Source: CAD feature listing. Evaluate the final solid. Frame: model axes, mm. A direction names the side the tool comes from. Round coordinates to 2 decimals unless told otherwise and drop trailing zeros. Order: outer loops, then holes, each group sorted by start corner. A loop starts at its lowest first (then second) coordinate and runs counter-clockwise, first axis right, second up. Notation, with made-up numbers: (61, 20) - (71, 20) arc R14 cw to (71, 31) - close; hole circle Ø3 at (-34, 8.25). An arc over 180 degrees is marked (long way). Use one line per item in the form item = value. Start each with the question number.
Q1. Ray query, line 1 (Y direction, x = -2, z = -1.75); line 2 (Y direction, x = -31, z = 2); line 3 (X direction, y = -9, z = -2.75). Return the intervals inside material, ascending. Write a range as [from, to].
Q2. Set-up query: faces 1 (the flat face through (-6, 22, 0)), 2 (the cylindrical face through (0, -13, 0)). Return all of +Z, -Z, +X, -X, +Y, -Y with unobstructed straight access to the full face (end or side cutting, diameter ignored); none if empty.
Q3. Draft query along Y for faces 3 (the cylindrical face through (-2.38, -10.74, -0.04)), 4 (the flat face through (-3, -12, -3.5)), 5 (the flat face through (22.41, -6.01, 0.05)). Return one class per face: released by +Y, released by -Y, zero draft, split by the parting line, or undercut.
Q4. Pin query (flat end, axial travel): pin 1 Ø4 at (x, z) = (-18, 0.5) entering from +Y; pin 2 Ø1 at (y, z) = (14.5, 2) entering from +X; pin 3 Ø1.5 at (x, z) = (-4.5, -2.5) entering from -Y; pin 4 Ø8 at (x, y) = (-10.5, 30) entering from -Z. Return the tip coordinate at first contact, or that it passes through.
Q5. Cut plane A-A, the plane x = 0. Return the cut outline in (y, z).
Q6. Cut plane C-C, the plane z = -1.5. Return the cut outline in (x, y), and give its area (3 significant figures).
Q7. Cut plane D-D, the plane y = 22. Return the cut outline in (x, z).
Q8. Cut plane B-B, the plane y = -16.5. Return the cut outline in (x, z), and give its area (3 significant figures).
from build123d import *

# Parameters (mm, degrees)
F0_R     = 11
F0_R_2   = 4
F1_DEPTH = 3.5
F2_SIZE  = 1


# Not quite as in the source:
# - a feature names something its author has since deleted; it is built from what else it names


with BuildPart() as f1:
    # F0 (on Top) → F1 (new body, symmetric)
    with BuildSketch(Plane.XY):
        with BuildLine():
            ThreePointArc((-6, 11.5325625947), (0, 13), (6, 11.5325625947))
            Line((6, 11.5325625947), (6, 33))
            ThreePointArc((6, 33), (0, 27), (-6, 33))
            Line((-6, 33), (-6, 11.5325625947))
        make_face()
        with BuildLine():
            ThreePointArc((-6.9874921777, -10.96243372), (-11.2583302492, -6.5), (-12.9874921777, -0.5701288746))
            Line((-12.9874921777, -0.5701288746), (-31.5788383249, -11.3038475773))
            ThreePointArc((-31.5788383249, -11.3038475773), (-25.5788383249, -11.3038475773), (-22.5788383249, -16.5))
            ThreePointArc((-22.5788383249, -16.5), (-23.3826859022, -19.5), (-25.5788383249, -21.6961524227))
            Line((-25.5788383249, -21.6961524227), (-6.9874921777, -10.96243372))
        make_face()
        with BuildLine():
            Line((31.5788383249, -11.3038475773), (12.9874921777, -0.5701288746))
            ThreePointArc((12.9874921777, -0.5701288746), (11.2583302492, -6.5), (6.9874921777, -10.96243372))
            Line((6.9874921777, -10.96243372), (25.5788383249, -21.6961524227))
            ThreePointArc((25.5788383249, -21.6961524227), (23.3826859022, -13.5), (31.5788383249, -11.3038475773))
        make_face()
        with BuildLine():
            ThreePointArc((12.9874921777, -0.5701288746), (12.9968726683, -0.2851330301), (13, 0))
            ThreePointArc((13, 0), (11.1130553854, 6.7453687816), (6, 11.5325625947))
            ThreePointArc((6, 11.5325625947), (0, 13), (-6, 11.5325625947))
            ThreePointArc((-6, 11.5325625947), (-11.2583302492, 6.5), (-12.9874921777, -0.5701288746))
            ThreePointArc((-12.9874921777, -0.5701288746), (-11.2583302492, -6.5), (-6.9874921777, -10.96243372))
            ThreePointArc((-6.9874921777, -10.96243372), (0, -13), (6.9874921777, -10.96243372))
            ThreePointArc((6.9874921777, -10.96243372), (11.2583302492, -6.5), (12.9874921777, -0.5701288746))
        make_face()
        Circle(F0_R, mode=Mode.SUBTRACT)
        with BuildLine():
            ThreePointArc((-6, 33), (0, 27), (6, 33))
            ThreePointArc((6, 33), (0, 39), (-6, 33))
        make_face()
        with Locations((0, 33)):
            Circle(F0_R_2, mode=Mode.SUBTRACT)
        with BuildLine():
            ThreePointArc((-22.5788383249, -16.5), (-25.5788383249, -11.3038475773), (-31.5788383249, -11.3038475773))
            ThreePointArc((-31.5788383249, -11.3038475773), (-33.7749907476, -19.5), (-25.5788383249, -21.6961524227))
            ThreePointArc((-25.5788383249, -21.6961524227), (-23.3826859022, -19.5), (-22.5788383249, -16.5))
        make_face()
        with Locations((-28.5788383249, -16.5)):
            Circle(F0_R_2, mode=Mode.SUBTRACT)
        with BuildLine():
            ThreePointArc((34.5788383249, -16.5), (33.7749907476, -13.5), (31.5788383249, -11.3038475773))
            ThreePointArc((31.5788383249, -11.3038475773), (23.3826859022, -13.5), (25.5788383249, -21.6961524227))
            ThreePointArc((25.5788383249, -21.6961524227), (31.5788383249, -21.6961524227), (34.5788383249, -16.5))
        make_face()
        with Locations((28.5788383249, -16.5)):
            Circle(F0_R_2, mode=Mode.SUBTRACT)
    extrude(amount=F1_DEPTH, both=True)

    # F2
    f2_edges = [f1.edges().sort_by_distance(p)[0] for p in [
        (-4, 33, 3.5),
        (-11, 0, 3.5),
        (-32.578838, -16.5, 3.5),
        (24.578838, -16.5, 3.5),
        (-32.578838, -16.5, -3.5),
        (-11, 0, -3.5),
        (24.578838, -16.5, -3.5),
        (-4, 33, -3.5),
    ]]
    chamfer(f2_edges, length=F2_SIZE)


solid = f1.part
Completed:
q1.line_1 = [-12.85, -10.82], [10.82, 29.54], [36.46, 38.66]
q1.line_2 = [-21.99, -19.68], [-13.32, -10.97]
q1.line_3 = [-27.59, -6.75], [6.75, 27.59]
q2.face_1 = +Z, -Z, -X, +Y
q2.face_2 = +Z, -Z, -Y
q3.face_3 = undercut
q3.face_4 = zero draft
q3.face_5 = released by +Y
q4.pin_1 = -2.31
q4.pin_2 = 6
q4.pin_3 = -12.45
q4.pin_4 = through
q5.outline = (-13, -3.5) - (-12, -3.5) - (-11, -2.5) - (-11, 2.5) - (-12, 3.5) - (-13, 3.5) - close; (11, -2.5) - (12, -3.5) - (28, -3.5) - (29, -2.5) - (29, 2.5) - (28, 3.5) - (12, 3.5) - (11, 2.5) - close; (37, -2.5) - (38, -3.5) - (39, -3.5) - (39, 3.5) - (38, 3.5) - (37, 2.5) - close
q6.outline = (-31.58, -11.3) arc R6 ccw to (-25.58, -21.7) - (-6.99, -10.96) arc R13 ccw to (6.99, -10.96) - (25.58, -21.7) arc R6 ccw to (31.58, -11.3) - (12.99, -0.57) arc R13 ccw to (6, 11.53) - (6, 33) arc R6 ccw to (-6, 33) - (-6, 11.53) arc R13 ccw to (-12.99, -0.57) - close; hole circle Ø8 at (-28.58, -16.5); hole circle Ø22 at (0, 0); hole circle Ø8 at (0, 33); hole circle Ø8 at (28.58, -16.5)
q6.area = 907 mm2
q7.outline = (-6, -3.5) - (6, -3.5) - (6, 3.5) - (-6, 3.5) - close
q8.outline = (-34.58, -3.5) - (-33.58, -3.5) - (-32.58, -2.5) - (-32.58, 2.5) - (-33.58, 3.5) - (-34.58, 3.5) - close; (-24.58, -2.5) - (-23.58, -3.5) - (-16.58, -3.5) - (-16.58, 3.5) - (-23.58, 3.5) - (-24.58, 2.5) - close; (16.58, -3.5) - (23.58, -3.5) - (24.58, -2.5) - (24.58, 2.5) - (23.58, 3.5) - (16.58, 3.5) - close; (32.58, -2.5) - (33.58, -3.5) - (34.58, -3.5) - (34.58, 3.5) - (33.58, 3.5) - (32.58, 2.5) - close
q8.area = 136 mm2
